from build123d import *

# Parameters (mm, degrees)
SKETCH1_R           = 11.25
BOSS_EXTRUDE1_DEPTH = 9.6
SKETCH2_R           = 3.625
BOSS_EXTRUDE2_DEPTH = 20
SKETCH3_R           = 6.7
BOSS_EXTRUDE3_DEPTH = 0.7
SKETCH4_R           = 0.875
BOSS_EXTRUDE4_DEPTH = 1.9
SKETCH5_R           = 2.9
CUT_EXTRUDE1_DEPTH  = 2
BOSS_EXTRUDE5_DEPTH = 27.65
CHAMFER1_SIZE2      = 0.577350269
CHAMFER1_SIZE       = 1


with BuildPart() as part:
    # Sketch1 → Boss-Extrude1 (new body)
    with BuildSketch(Plane(origin=(0, 0, 0), x_dir=(0, 0, -1), z_dir=(1, 0, 0))):
        Circle(SKETCH1_R)
    extrude(amount=-BOSS_EXTRUDE1_DEPTH)

    # Sketch2 → Boss-Extrude2 (add)
    with BuildSketch(Plane(origin=(0, 0, 0), x_dir=(1, 0, 0), z_dir=(0, 1, 0))):
        with Locations(Location((-4.8, -7.625, 0), (0, 0, 270))):
            Circle(SKETCH2_R)
    extrude(amount=BOSS_EXTRUDE2_DEPTH)

    # Sketch3 → Boss-Extrude3 (add)
    with BuildSketch(Plane(origin=(0, 0, 0), x_dir=(0, 0, -1), z_dir=(1, 0, 0))):
        Circle(SKETCH3_R)
    extrude(amount=BOSS_EXTRUDE3_DEPTH)

    # Sketch4 → Boss-Extrude4 (add)
    with BuildSketch(Plane(origin=(0, 0, 0), x_dir=(0, 0, -1), z_dir=(1, 0, 0))):
        with Locations(Location((0, 8.833459119, 0), (0, 0, 180))):
            Circle(SKETCH4_R)
        with Locations(Location((7.65, -4.416729559, 0), (0, 0, 180))):
            Circle(SKETCH4_R)
        with Locations(Location((-7.65, -4.416729559, 0), (0, 0, 180))):
            Circle(SKETCH4_R)
    extrude(amount=BOSS_EXTRUDE4_DEPTH)

    # Sketch5 → Cut-Extrude1 (cut)
    with BuildSketch(Plane(origin=(0.7, 0, 0), x_dir=(0, 0, -1), z_dir=(1, 0, 0))):
        Circle(SKETCH5_R)
    extrude(amount=-CUT_EXTRUDE1_DEPTH, mode=Mode.SUBTRACT)

    # Sketch7 → Revolve1 (revolve)
    with BuildSketch(Plane.XY):
        Polygon((-9.6, 0), (-9.6, 11.25), (-41.3, 11.75), (-41.3, 0), align=None)
    revolve(axis=Axis((-9.6, 0, 0), (-1, 0, 0)))

    # Sketch8 → Boss-Extrude5 (add)
    with BuildSketch(Plane(origin=(-9.6, 0, 0), x_dir=(0, 0, -1), z_dir=(1, 0, 0))):
        Polygon((-10, -11.75), (10, -11.75), (10, -10.5), (3.216946356, -8.409910385), (-3.216946356, -8.409910385), (-10, -10.5), align=None)
    extrude(amount=-BOSS_EXTRUDE5_DEPTH)

    # Chamfer1
    chamfer1_edges = [part.edges().sort_by_distance(p)[0] for p in [
        (-4.8, 20, 4),
    ]]
    chamfer(chamfer1_edges, length=CHAMFER1_SIZE, length2=CHAMFER1_SIZE2)


solid = part.part
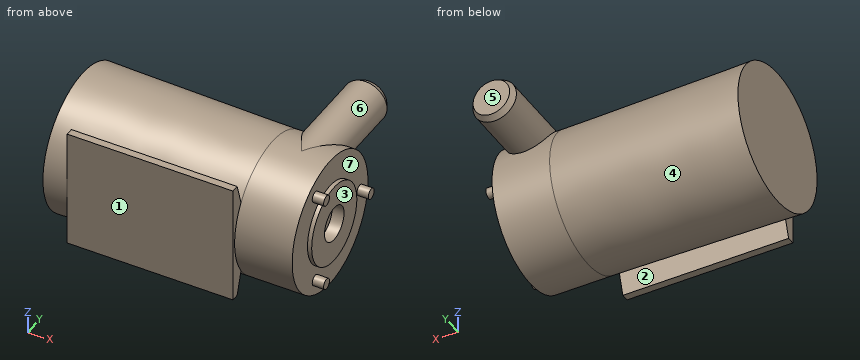
Source: CAD feature listing. Evaluate the final solid. Frame: model axes, mm. Face numbers are marked on the shaded views. A direction names the side the tool comes from. Round coordinates to 2 decimals unless told otherwise and drop trailing zeros. Order: outer loops, then holes, each group sorted by start corner. A loop starts at its lowest first (then second) coordinate and runs counter-clockwise, first axis right, second up. Notation, with made-up numbers: (85, 77.5) - (129, 77.5) arc R19 ccw to (129, 104.5) - close; hole circle Ø7 at (32, -31). An arc over 180 degrees is marked (long way). Use a Markdown table: item, result. Add a question column.
1. Section query C-C (x = -17). Return the cut outline in (y, z), then the cut area to 3 significant figures.
2. Section query B-B (y = 15). Return the cut outline in (x, z) (3 decimals), then the cut area to 3 significant figures.
3. First-contact query: pin 1 (4 mm diameter, centred on x = -4.5, z = -1, fed in from -Y); pin 2 (7 mm diameter, centred on y = -4, z = 2, fed in from +X); pin 3 (1.4 mm diameter, centred on x = -29, y = -11, fed in from +Z). Flat tips, straight axial feed; report the tip coordinate or a pass-through.
4. Line query: probe 1 along Y at (x, z) = (0.2, 0); probe 2 along Y at (x, z) = (-0.7, 0); probe 3 along X at (y, z) = (-3.5, -6.75). Output: solid intervals per line, ascending.
5. Section query A-A (x = -4.8). Return the cut outline in (y, z).
6. Set-up query: the marked faces 5, 6 and 7. Return all of +Z, -Z, +X, -X, +Y, -Y with unobstructed straight access to the full face (end or side cutting, diameter ignored); none if empty.
7. Mould query, pull axis Y, two halves, no side actions, for the marked faces 1, 2, 3 and 4. Classes: +Y half, -Y half, draft (parallel to the pull), parting line (faces both ways), or undercut.
Derived:
| question | item | result |
|---|---|---|
| 1 | outline | (-11.75, -10) - (-10.5, -10) - (-9.39, -6.4) arc R11.37 ccw (long way) to (-9.39, 6.4) - (-10.5, 10) - (-11.75, 10) - close |
| 1 | area | 432 mm2 |
| 2 | outline | circle Ø7.25 at (-4.8, 7.625) |
| 2 | area | 41.3 mm2 |
| 3 | pin 1 | y = -11.25 |
| 3 | pin 2 | x = 0.7 |
| 3 | pin 3 | z = 10 |
| 4 | probe 1 | -6.7 to -2.9, 2.9 to 6.7, 7.96 to 9.71 |
| 4 | probe 2 | -11.25 to -2.9, 2.9 to 11.25 |
| 4 | probe 3 | -41.3 to 0 |
| 5 | outline | (0, 11.25) arc R11.25 ccw (long way) to (10.51, 4) - (19, 4) - (20, 4.58) - (20, 10.67) - (19, 11.25) - close |
| 6 | face 5 | +Z, -Z, +X, -X, +Y |
| 6 | face 6 | +Y |
| 6 | face 7 | +X |
| 7 | face 1 | -Y half |
| 7 | face 2 | undercut |
| 7 | face 3 | draft |
| 7 | face 4 | undercut |
